Part model, mm, in its own coordinate system. Face numbers are marked on the shaded views. Give positions to 0.01 mm unless a question says otherwise; leave off trailing zeros. Write each loop counter-clockwise with the first axis right and the second up, starting at its lowest first coordinate (ties: lowest second). Pieces come first, ordered by that corner, then holes.
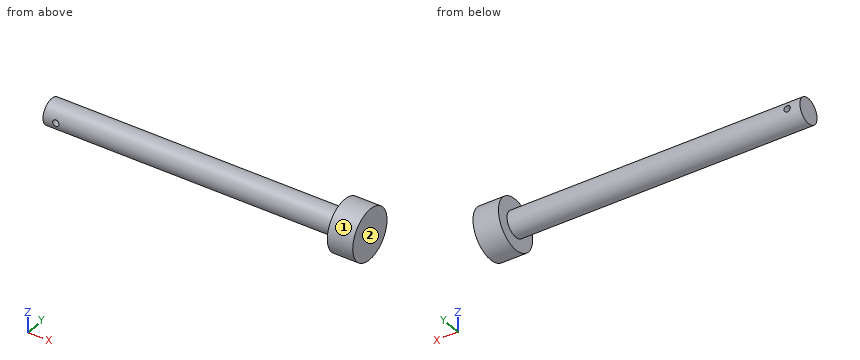
from build123d import *

# Parameters (mm, degrees)
SKETCH1_R               = 16
BOSS_EXTRUDE1_DEPTH     = 16
SKETCH2_R               = 8
BOSS_EXTRUDE2_DEPTH     = 200
CUT_EXTRUDE2_DEPTH      = 186.38608362
CUT_EXTRUDE2_DEPTH_BACK = 186.38608362
SKETCH3_R               = 2


with BuildPart() as part:
    # Sketch1 → Boss-Extrude1 (new body)
    with BuildSketch(Plane(origin=(0, 0, 0), x_dir=(0, 0, -1), z_dir=(1, 0, 0))):
        Circle(SKETCH1_R)
    extrude(amount=BOSS_EXTRUDE1_DEPTH)

    # Sketch2 → Boss-Extrude2 (add)
    with BuildSketch(Plane(origin=(16, 0, 0), x_dir=(0, 0, -1), z_dir=(1, 0, 0))):
        Circle(SKETCH2_R)
    extrude(amount=-BOSS_EXTRUDE2_DEPTH)

    # Sketch3 → Cut-Extrude2 (cut, two sides: drawn at the far end of the back side and taken through both)
    with BuildSketch(Plane(origin=(0, 0, 0), x_dir=(1, 0, 0), z_dir=(0, 1, 0)).offset(-CUT_EXTRUDE2_DEPTH_BACK)):
        with Locations(Location((-176, 0, 0), (0, 0, 270))):
            Circle(SKETCH3_R)
    extrude(amount=CUT_EXTRUDE2_DEPTH + CUT_EXTRUDE2_DEPTH_BACK, mode=Mode.SUBTRACT)


solid = part.part
1) Saw through at C-C (x = -28). Write the cut outline in (y, z).
Check result:
outline: circle Ø16 at (0, 0)
2) Saw through at A-A (z = 0). Write the cut outline in (x, y).
Check result:
outline: (-184, -8) - (-178, -8) - (-178, 8) - (-184, 8) - close; (-174, -8) - (0, -8) - (0, -16) - (16, -16) - (16, 16) - (0, 16) - (0, 8) - (-174, 8) - close
3) Saw through at D-D (y = 10.5). Write the cut outline in (x, z), and give its area (3 significant figures).
Check result:
outline: (0, -12.07) - (16, -12.07) - (16, 12.07) - (0, 12.07) - close
area: 386 mm2
4) Mould opens along Y. For the marked faces 1 and 2 say: +Y half, -Y half, draft (parallel to the pull), parting line (faces both ways), or undercut.
Check result:
face 1: parting line
face 2: draft
5) Saw through at B-B (y = 0). Write the cut outline in (x, z).
Check result:
outline: (-184, -8) - (0, -8) - (0, -16) - (16, -16) - (16, 16) - (0, 16) - (0, 8) - (-184, 8) - close; hole circle Ø4 at (-176, 0)
6) Flat gauge pins, fed straight in: P1, Ø1, axis at y = 10, z = 6, coming from the -X side; P2, Ø12, axis at x = -128, y = 8.5, coming from the +Z side; P3, Ø5, axis at x = -109.5, z = -2.5, coming from the +Y side. Where does each tip first touch, or does it go through?
Check result:
P1: stops at x = 0
P2: stops at z = 7.6
P3: stops at y = 8
7) Drill centre lines: L1, parallel to X at y = 4, z = 0; L2, parallel to Z at x = -176, y = -0.25; L3, parallel to X at y = 7, z = 4.5. Where is each one in solid material? Low to high.
Check result:
L1: x = -184 to -178, -174 to 16
L2: z = -8 to -2, 2 to 8
L3: x = 0 to 16
